from build123d import *

# Parameters (mm, degrees)
F0_W     = 100
F0_H     = 50
F1_DEPTH = 10
F2_W     = 100
F2_H     = 5
F3_DEPTH = 18.6
F4_R     = 2.5
F5_DEPTH = 5.001


with BuildPart() as f1:
    # F0 (on Top) → F1 (new body)
    with BuildSketch(Plane.XY):
        with Locations((-0.122877, -25)):
            Rectangle(F0_W, F0_H)
    extrude(amount=F1_DEPTH)

    # F2 (on face) → F3 (join)
    with BuildSketch(Plane.XY.offset(10)):
        with Locations((-0.122877, -2.5)):
            Rectangle(F2_W, F2_H)
    extrude(amount=F3_DEPTH)

    # F4 (on face) → F5 (cut, through all)
    with BuildSketch(Plane.XZ.offset(5)):
        with Locations((20, 25)):
            Circle(F4_R)
        with Locations((-20, 25)):
            Circle(F4_R)
    extrude(amount=-F5_DEPTH, mode=Mode.SUBTRACT)


solid = f1.part
Source: CAD feature listing. Evaluate the final solid. Frame: model axes, mm. A direction names the side the tool comes from. Round coordinates to 2 decimals unless told otherwise and drop trailing zeros. Order: outer loops, then holes, each group sorted by start corner. A loop starts at its lowest first (then second) coordinate and runs counter-clockwise, first axis right, second up. Notation, with made-up numbers: (6.5, -16) - (27.5, -16) arc R32 ccw to (27.5, 11) - close; hole circle Ø8 at (8, 41.5). An arc over 180 degrees is marked (long way). Use a Markdown table: item, result. Add a question column.
1. Section query B-B (x = 20). Return the cut outline in (y, z).
2. Mould query, pull axis X, two halves, no side actions, for faces 3 (the flat face through (-1, -27, 10)), 4 (the cylindrical face through (18.16, -2.54, 26.69)), 5 (the flat face through (-50.123, -20, 8)). Classes: +X half, -X half, draft (parallel to the pull), parting line (faces both ways), or undercut.
3. Set-up query: faces 1 (the flat face through (-1, -5, 19)), 2 (the flat face through (-1, -2, 28.6)). Return all of +Z, -Z, +X, -X, +Y, -Y with unobstructed straight access to the full face (end or side cutting, diameter ignored); none if empty.
4. Line query: probe 1 along Z at (x, y) = (20, -1.7); probe 2 along Z at (x, y) = (4.5, -33.5); probe 3 along Y at (x, z) = (-46, 23). Output: solid intervals per line, ascending.
5. First-contact query: pin 1 (15 mm diameter, centred on x = 16.5, z = 23.5, fed in from -Y); pin 2 (4 mm diameter, centred on x = -20, z = 25, fed in from -Y). Flat tips, straight axial feed; report the tip coordinate or a pass-through.
6. Section query A-A (z = 25). Return the cut outline in (x, y).
7. Section query D-D (y = -6). Return the cut outline in (x, z), then the cut area to 3 significant figures.
8. Section query C-C (x = -7). Return the cut outline in (y, z).
Derived:
| question | item | result |
|---|---|---|
| 1 | outline | (-50, 0) - (0, 0) - (0, 22.5) - (-5, 22.5) - (-5, 10) - (-50, 10) - close; (-5, 27.5) - (0, 27.5) - (0, 28.6) - (-5, 28.6) - close |
| 2 | face 3 | draft |
| 2 | face 4 | undercut |
| 2 | face 5 | -X half |
| 3 | face 1 | +Z, +X, -X, -Y |
| 3 | face 2 | +Z, +X, -X, +Y, -Y |
| 4 | probe 1 | 0 to 22.5, 27.5 to 28.6 |
| 4 | probe 2 | 0 to 10 |
| 4 | probe 3 | -5 to 0 |
| 5 | pin 1 | y = -5 |
| 5 | pin 2 | through |
| 6 | outline | (-50.12, -5) - (-22.5, -5) - (-22.5, 0) - (-50.12, 0) - close; (-17.5, -5) - (17.5, -5) - (17.5, 0) - (-17.5, 0) - close; (22.5, -5) - (49.88, -5) - (49.88, 0) - (22.5, 0) - close |
| 7 | outline | (-50.12, 0) - (49.88, 0) - (49.88, 10) - (-50.12, 10) - close |
| 7 | area | 1,000 mm2 |
| 8 | outline | (-50, 0) - (0, 0) - (0, 28.6) - (-5, 28.6) - (-5, 10) - (-50, 10) - close |
